Can you work these out from the drawing? Everything is in mm from the part's minimum corner. A direction names the side the tool comes from. Coordinates: 2 decimals unless noted, no trailing zeros. Order: outer loops, then holes, each group sorted by start corner. A loop starts at its lowest first (then second) coordinate and runs counter-clockwise, first axis right, second up. Notation, with made-up numbers: (14.25, -30.5) - (62.25, -30.5) arc R34 cw to (62.25, 6.5) - close; hole circle Ø11 at (44, 72.5). An arc over 180 degrees is marked (long way). Use a Markdown table: item, result. Add a question column.
(1) We'd pull the mould along X, two halves only. Please class the marked faces 1, 2, 3 and 4: pulls with the +X half, pulls with the -X half, needs draft (parallel to the pull), parting line crosses it, or undercut.
(2) I want a section at B-B (x = 145). List the corners of the cut face in (y, z) for me.
(3) I want a section at A-A (z = 6.35). List the corners of the cut face in (x, y) for me, and give its area (3 significant figures).
(4) If I drill on L1, parallel to X at y = 25, z = 6.35; L2, parallel to X at y = 13, z = 58.5; L3, parallel to Y at x = 48, z = 16, over which ranges is the centre line in solid material (lowest first)? Write a range as [from, to].
(5) I want a section at C-C (z = 49.5). List the corners of the cut face in (x, y) for me, and give its area (3 significant figures).
(6) On a 3-axis mill with a long thin cutter (end or side, diameter ignored), from which of +Z, -Z, +X, -X, +Y, -Y can I reach the whole of each face in a straight line? I mean the marked faces 5, 6 and 7. Say none if no direction works.
(7) For pin 1 Ø10 at (y, z) = (12.5, 39.5) entering from -X; pin 2 Ø19 at (x, z) = (143.5, 43.5) entering from +Y; pin 3 Ø8 at (x, z) = (98.425, 6.35) entering from +Y; pin 4 Ø10 at (x, y) = (8, 27.5) entering from +Z, each with a flat end and sliding along its axis, tell me the tip position at first contact or that it passes through.
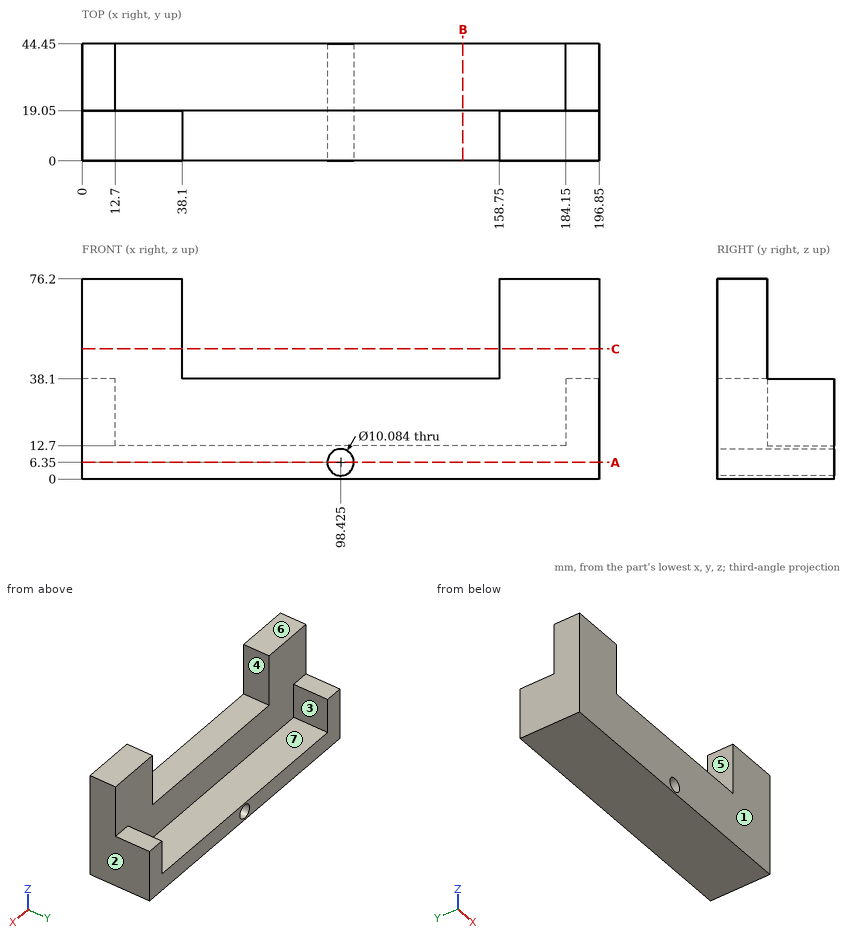
Answers follow:
| question | item | result |
|---|---|---|
| 1 | face 1 | needs draft |
| 1 | face 2 | pulls with the +X half |
| 1 | face 3 | undercut |
| 1 | face 4 | undercut |
| 2 | outline | (0, 0) - (44.45, 0) - (44.45, 12.7) - (19.05, 12.7) - (19.05, 38.1) - (0, 38.1) - close |
| 3 | outline | (0, 0) - (93.38, 0) - (93.38, 44.45) - (0, 44.45) - close; (103.47, 0) - (196.85, 0) - (196.85, 44.45) - (103.47, 44.45) - close |
| 3 | area | 8,300 mm² |
| 4 | L1 | x = [0, 93.38], [103.47, 196.85] |
| 4 | L2 | x = [0, 38.1], [158.75, 196.85] |
| 4 | L3 | y = [0, 19.05] |
| 5 | outline | (0, 0) - (38.1, 0) - (38.1, 19.05) - (0, 19.05) - close; (158.75, 0) - (196.85, 0) - (196.85, 19.05) - (158.75, 19.05) - close |
| 5 | area | 1,450 mm² |
| 6 | face 5 | +Z, +Y, -Y |
| 6 | face 6 | +Z, +X, -X, +Y, -Y |
| 6 | face 7 | +Z, +Y |
| 7 | pin 1 | stops at x = 0 |
| 7 | pin 2 | stops at y = 19.05 |
| 7 | pin 3 | passes through |
| 7 | pin 4 | stops at z = 38.1 |
